Verification items for the finished model (mm, model axes). A direction names the side the tool comes from. Give positions to 0.01 mm unless a question says otherwise; leave off trailing zeros. Order: outer loops, then holes, each group sorted by start corner. A loop starts at its lowest first (then second) coordinate and runs counter-clockwise, first axis right, second up.
from build123d import *

# Parameters (mm, degrees)
SKETCH1_W           = 35
SKETCH1_H           = 40
BOSS_EXTRUDE1_DEPTH = 6
CUT_EXTRUDE1_DEPTH  = 35
FILLET4_R           = 0.3
CUT_EXTRUDE4_DEPTH  = 20
CHAMFER1_SIZE       = 0.1
SKETCH10_W          = 20.487766081
SKETCH10_H          = 1.5
CUT_EXTRUDE8_DEPTH  = 45.070965499
CUT_EXTRUDE9_DEPTH  = 1.75
CUT_EXTRUDE10_DEPTH = 1.25
SKETCH13_W          = 15
SKETCH13_H          = 20
CUT_EXTRUDE11_DEPTH = 3.5
SKETCH14_W          = 15
SKETCH14_H          = 1.5
SKETCH14_W_2        = 3.5
SKETCH14_H_2        = 2
BOSS_EXTRUDE2_DEPTH = 1.5
FILLET5_R           = 1
SKETCH15_R          = 0.9
BOSS_EXTRUDE3_DEPTH = 1.5
BOSS_EXTRUDE4_START = 7
SKETCH15_3_R        = 0.9
BOSS_EXTRUDE4_DEPTH = 1
SKETCH15_4_R        = 0.9
BOSS_EXTRUDE5_DEPTH = 8


with BuildPart() as part:
    # Sketch1 → Boss-Extrude1 (new body)
    with BuildSketch(Plane.XY):
        Rectangle(SKETCH1_W, SKETCH1_H)
    extrude(amount=BOSS_EXTRUDE1_DEPTH)

    # Sketch2 → Cut-Extrude1 (cut)
    with BuildSketch(Plane.XZ.offset(20)):
        Polygon((-10.767949192, 6), (-9.035898385, 3), (-15.5, 3), (-13.767949192, 6), align=None)
    extrude(amount=-CUT_EXTRUDE1_DEPTH, mode=Mode.SUBTRACT)

    # Fillet4
    fillet4_edges = [part.edges().sort_by_distance(p)[0] for p in [
        (-13.767949192, -2.5, 6),
        (-10.767949192, -2.5, 6),
    ]]
    fillet(fillet4_edges, radius=FILLET4_R)

    # Sketch5 → Cut-Extrude4 (cut)
    with BuildSketch(Plane.XZ.offset(20)):
        Polygon((-4.882308546, 6), (-4.016283143, 4.5), (-7.24833395, 4.5), (-6.382308546, 6), align=None)
    extrude(amount=-CUT_EXTRUDE4_DEPTH, mode=Mode.SUBTRACT)

    # Chamfer1
    chamfer1_edges = [part.edges().sort_by_distance(p)[0] for p in [
        (-6.382308546, -10, 6),
        (-4.882308546, -10, 6),
    ]]
    chamfer(chamfer1_edges, length=CHAMFER1_SIZE)

    # Sketch10 → Cut-Extrude8 (cut, through all)
    with BuildSketch(Plane.XZ.offset(20)):
        with Locations((7.256116959, 0.75)):
            Rectangle(SKETCH10_W, SKETCH10_H)
    extrude(amount=-CUT_EXTRUDE8_DEPTH, mode=Mode.SUBTRACT)

    # Sketch11 → Cut-Extrude9 (cut, symmetric)
    with BuildSketch(Plane(origin=(-12.267949192, 0, 0), x_dir=(0, 0, -1), z_dir=(1, 0, 0))):
        Polygon((-3, -19), (-3, -6), (-2.3, -19), align=None)
    extrude(amount=CUT_EXTRUDE9_DEPTH, both=True, mode=Mode.SUBTRACT)

    # Sketch12 → Cut-Extrude10 (cut, symmetric)
    with BuildSketch(Plane(origin=(-5.632308546, 0, 0), x_dir=(0, 0, -1), z_dir=(1, 0, 0))):
        Polygon((-4.5, -19.2), (-4.5, -11.198963388), (-3.8, -19.2), align=None)
    extrude(amount=CUT_EXTRUDE10_DEPTH, both=True, mode=Mode.SUBTRACT)

    # Sketch13 → Cut-Extrude11 (cut)
    with BuildSketch(Plane.XY.offset(6)):
        with Locations((5.717691454, -7)):
            Rectangle(SKETCH13_W, SKETCH13_H)
    extrude(amount=-CUT_EXTRUDE11_DEPTH, mode=Mode.SUBTRACT)

    # Sketch14 → Boss-Extrude2 (add)
    with BuildSketch(Plane.XY.offset(6)):
        with Locations((5.717691454, -16.25)):
            Rectangle(SKETCH14_W, SKETCH14_H)
        with Locations((-0.032308546, 2)):
            Rectangle(SKETCH14_W_2, SKETCH14_H_2)
        with Locations((11.467691454, 2)):
            Rectangle(SKETCH14_W_2, SKETCH14_H_2)
    extrude(amount=-BOSS_EXTRUDE2_DEPTH)

    # Fillet5
    fillet5_edges = [part.edges().sort_by_distance(p)[0] for p in [
        (1.717691454, 1, 5.25),
        (9.717691454, 1, 5.25),
    ]]
    fillet(fillet5_edges, radius=FILLET5_R)

    # Sketch15 → Boss-Extrude3 (add)
    # profile 1 of 2: a face of its own
    with BuildSketch(Plane(origin=(0, 0, 0), x_dir=(0, 0, -1), z_dir=(1, 0, 0))):
        with BuildLine():
            Line((2.922618262, 16.125083661), (-1.5, 14.062782897))
            Line((-1.5, 14.062782897), (-1.5, 20))
            Line((-1.5, 20), (2.922618262, 17.937699235))
            ThreePointArc((2.922618262, 17.937699235), (3.5, 17.031391448), (2.922618262, 16.125083661))
        make_face()
        with Locations((2.5, 17.031391448)):
            Circle(SKETCH15_R, mode=Mode.SUBTRACT)
    # profile 2 of 2: a face of its own
    with BuildSketch(Plane(origin=(0, 0, 0), x_dir=(0, 0, -1), z_dir=(1, 0, 0))):
        with BuildLine():
            ThreePointArc((2.922618262, -2.062300765), (3.5, -2.968608552), (2.922618262, -3.874916339))
            Line((2.922618262, -3.874916339), (-1.5, -5.937217103))
            Line((-1.5, -5.937217103), (-1.5, 0))
            Line((-1.5, 0), (2.922618262, -2.062300765))
        make_face()
        with Locations((2.5, -2.968608552)):
            Circle(SKETCH15_R, mode=Mode.SUBTRACT)
    extrude(amount=BOSS_EXTRUDE3_DEPTH)

    # Sketch15<3> → Boss-Extrude4 (add)
    # profile 1 of 2: a face of its own
    with BuildSketch(Plane(origin=(0, 0, 0), x_dir=(0, 0, -1), z_dir=(1, 0, 0)).offset(BOSS_EXTRUDE4_START)):
        with BuildLine():
            ThreePointArc((2.922618262, -2.062300765), (3.5, -2.968608552), (2.922618262, -3.874916339))
            Line((2.922618262, -3.874916339), (-1.5, -5.937217103))
            Line((-1.5, -5.937217103), (-1.5, 0))
            Line((-1.5, 0), (2.922618262, -2.062300765))
        make_face()
        with Locations((2.5, -2.968608552)):
            Circle(SKETCH15_3_R, mode=Mode.SUBTRACT)
    # profile 2 of 2: a face of its own
    with BuildSketch(Plane(origin=(0, 0, 0), x_dir=(0, 0, -1), z_dir=(1, 0, 0)).offset(BOSS_EXTRUDE4_START)):
        with BuildLine():
            Line((2.922618262, 16.125083661), (-1.5, 14.062782897))
            Line((-1.5, 14.062782897), (-1.5, 20))
            Line((-1.5, 20), (2.922618262, 17.937699235))
            ThreePointArc((2.922618262, 17.937699235), (3.5, 17.031391448), (2.922618262, 16.125083661))
        make_face()
        with Locations((2.5, 17.031391448)):
            Circle(SKETCH15_3_R, mode=Mode.SUBTRACT)
    extrude(amount=BOSS_EXTRUDE4_DEPTH)

    # Sketch15<4> → Boss-Extrude5 (add)
    with BuildSketch(Plane(origin=(0, 0, 0), x_dir=(0, 0, -1), z_dir=(1, 0, 0))):
        with Locations((2.5, 17.031391448)):
            Circle(SKETCH15_4_R)
        with Locations((2.5, -2.968608552)):
            Circle(SKETCH15_4_R)
    extrude(amount=BOSS_EXTRUDE5_DEPTH)


solid = part.part
(1) Section check A-A, the plane y = 9. Enter the section's corners in (x, z).
Solved:
outline: (-17.5, 0) - (-2.99, 0) - (-2.99, 1.5) - (17.5, 1.5) - (17.5, 6) - (-10.25, 6) arc R0.3 ccw to (-10.51, 5.55) - (-9.04, 3) - (-15.5, 3) - (-14.03, 5.55) arc R0.3 ccw to (-14.29, 6) - (-17.5, 6) - close
(2) Section check D-D, the plane x = -11. Enter the section's corners in (y, z).
Solved:
outline: (-20, 0) - (20, 0) - (20, 6) - (15, 6) - (15, 3) - (-6, 3) - (-19, 2.3) - (-19, 3) - (-20, 3) - close
(3) Release check for a two-part mould opening along Z. For faces 4 (the flat face through (-2.988, 0, 1)), 5 (the cylindrical face through (7.5, -3, -3.5)), 6 (the flat face through (6, 3, 4)) record: pulls with the +Z half, pulls with the -Z half, needs draft (parallel to the pull), parting line crosses it, or undercut.
Solved:
face 4: needs draft
face 5: pulls with the -Z half
face 6: undercut
(4) Scan lines: line 1 (Y direction, x = 0, z = 4); line 2 (X direction, y = -10, z = 3.25); line 3 (Z direction, x = 2, y = -3). Record each from-to range of solid material in increasing order.
Solved:
line 1: y = -20 to -17, 3 to 20
line 2: x = -17.5 to -15.36, -9.18 to -1.78, 13.22 to 17.5
line 3: z = -3.4 to -1.6, 1.5 to 2.5
(5) Section check C-C, the plane z = -0.75. Enter the section's corners in (x, y), then the cut area to 3 significant figures.
Solved:
outline: (0, -4.89) - (1.5, -4.89) - (1.5, -1.05) - (0, -1.05) - close; (0, 15.11) - (1.5, 15.11) - (1.5, 18.95) - (0, 18.95) - close; (7, -4.89) - (8, -4.89) - (8, -1.05) - (7, -1.05) - close; (7, 15.11) - (8, 15.11) - (8, 18.95) - (7, 18.95) - close
area: 19.2 mm2
(6) Set-up check for faces 1 (the flat face through (-1, 1, 5)), 2 (the flat face through (0, 2, 4.5)), 3 (the flat face through (7.493, -4.892, -0.742)): record each of +Z, -Z, +X, -X, +Y, -Y from which the full face is reachable in a straight line by a thin tool's end or side.
Solved:
face 1: +Z
face 2: none
face 3: -Z, +X, -Y
(7) Go/stop test with flat-tipped pins: pin 1 (1.5 mm diameter, centred on x = 8, z = -2, fed in from +Y); pin 2 (12 mm diameter, centred on x = -11, y = -14.5, fed in from -Z); pin 3 (4 mm diameter, centred on y = -4, z = -2, fed in from +X). Record where each tip stops, or that it passes through.
Solved:
pin 1: stops at y = 18.72
pin 2: stops at z = 0
pin 3: stops at x = 8
(8) Section check B-B, the plane x = -5.5. Enter the section's corners in (y, z), then the cut area to 3 significant figures.
Solved:
outline: (-20, 0) - (20, 0) - (20, 6) - (0, 6) - (0, 4.5) - (-11.2, 4.5) - (-19.2, 3.8) - (-19.2, 4.5) - (-20, 4.5) - close
area: 207 mm2
